from build123d import *

# Parameters (mm, degrees)
ESQUISSE3_R        = 9
BOSS_EXTRU_1_DEPTH = 5
ESQUISSE4_W        = 10
ESQUISSE4_H        = 3
ESQUISSE4_W_2      = 35
BOSS_EXTRU_2_DEPTH = 20


with BuildPart() as part:
    # Esquisse3 → Boss.-Extru.1 (new body)
    with BuildSketch(Plane(origin=(0, 0, 0), x_dir=(1, 0, 0), z_dir=(0, 1, 0))):
        with BuildLine():
            Line((-42.049920388, -18.295081967), (-42.049920388, 31.704918033))
            ThreePointArc((-42.049920388, 31.704918033), (-39.120988199, 38.775985845), (-32.049920388, 41.704918033))
            Line((-32.049920388, 41.704918033), (17.950079612, 41.704918033))
            ThreePointArc((17.950079612, 41.704918033), (25.021147424, 38.775985845), (27.950079612, 31.704918033))
            Line((27.950079612, 31.704918033), (27.950079612, -15.295081967))
            Line((27.950079612, -15.295081967), (52.950079612, -15.295081967))
            Line((52.950079612, -15.295081967), (52.950079612, -18.295081967))
            Line((52.950079612, -18.295081967), (17.950079612, -18.295081967))
            Line((17.950079612, -18.295081967), (17.950079612, 11.704918033))
            Line((17.950079612, 11.704918033), (-32.049920388, 11.704918033))
            Line((-32.049920388, 11.704918033), (-32.049920388, -18.295081967))
            Line((-32.049920388, -18.295081967), (-42.049920388, -18.295081967))
        make_face()
        with Locations((-20.049920388, 26.704918033)):
            Circle(ESQUISSE3_R, mode=Mode.SUBTRACT)
        with Locations((5.950079612, 26.704918033)):
            Circle(ESQUISSE3_R, mode=Mode.SUBTRACT)
    extrude(amount=BOSS_EXTRU_1_DEPTH)

    # Esquisse4 → Boss.-Extru.2 (add)
    with BuildSketch(Plane(origin=(0, 5, 0), x_dir=(1, 0, 0), z_dir=(0, 1, 0))):
        with Locations((-37.049920388, -16.795081967)):
            Rectangle(ESQUISSE4_W, ESQUISSE4_H)
        with Locations((35.450079612, -16.795081967)):
            Rectangle(ESQUISSE4_W_2, ESQUISSE4_H)
    extrude(amount=-BOSS_EXTRU_2_DEPTH)


solid = part.part
Input: part model. Units: mm. Frame: model coordinates. A direction names the side the tool comes from. Round coordinates to 2 decimals unless told otherwise and drop trailing zeros. Write each loop counter-clockwise with the first axis right and the second up, starting at its lowest first coordinate (ties: lowest second). Pieces come first, ordered by that corner, then holes.
1) Ray query, L1, parallel to X at y = 3.25, z = -6.5; L2, parallel to Y at x = -11, z = -27.5; L3, parallel to Z at x = 29.5, y = -4.5. Return the intervals inside material, ascending.
2) Contact query for flat-ended pins moving along their axis: P1, Ø8, axis at x = -35.5, y = -5.5, coming from the -Z side; P2, Ø5, axis at y = 2.5, z = 3, coming from the +X side; P3, Ø4, axis at x = -1.5, y = 1.5, coming from the +Z side. Output: stop coordinate, or through.
3) Cut plane A-A (y = -6.25). Return the cut outline in (x, z).
4) Cut plane D-D (x = 26). Return the cut outline in (y, z).
5) Cut plane B-B (z = 5.5). Return the cut outline in (x, y), then the cut area to 3 significant figures.
6) Cut plane C-C (y = 1). Return the cut outline in (x, z).
7) Draft query along X for faces 4 (the flat face through (17.95, 1, 6)), 5 (the flat face through (-37, -7, 15.295)), 6 (the flat face through (27.95, 2, -9)). Return one class per face: pulls with the +X half, pulls with the -X half, needs draft (parallel to the pull), parting line crosses it, or undercut.
8) Reachability of faces 1 (the flat face through (-32.05, 0.2, 6.7)), 2 (the flat face through (-37, -5, 18.295)), 3 (the flat face through (-7, 0, -20)) from +Z, -Z, +X, -X, +Y, -Y: full face, straight path, thin tool, end or side. Return the list, or none.
Geometry says:
1. L1: x = -42.05 to -32.05, 17.95 to 27.95
1. L2: y = 0 to 5
1. L3: z = 15.3 to 18.3
2. P1: stops at z = 15.3
2. P2: stops at x = 27.95
2. P3: stops at z = -11.7
3. outline: (-42.05, 15.3) - (-32.05, 15.3) - (-32.05, 18.3) - (-42.05, 18.3) - close; (17.95, 15.3) - (52.95, 15.3) - (52.95, 18.3) - (17.95, 18.3) - close
4. outline: (-15, 15.3) - (0, 15.3) - (0, -37.64) - (5, -37.64) - (5, 18.3) - (-15, 18.3) - close
5. outline: (-42.05, 0) - (-32.05, 0) - (-32.05, 5) - (-42.05, 5) - close; (17.95, 0) - (27.95, 0) - (27.95, 5) - (17.95, 5) - close
5. area: 100 mm2
6. outline: (-42.05, -31.7) arc R10 ccw to (-32.05, -41.7) - (17.95, -41.7) arc R10 ccw to (27.95, -31.7) - (27.95, 15.3) - (52.95, 15.3) - (52.95, 18.3) - (17.95, 18.3) - (17.95, -11.7) - (-32.05, -11.7) - (-32.05, 18.3) - (-42.05, 18.3) - close; hole circle Ø18 at (-20.05, -26.7); hole circle Ø18 at (5.95, -26.7)
7. face 4: undercut
7. face 5: needs draft
7. face 6: pulls with the +X half
8. face 1: +Z, +Y, -Y
8. face 2: +Z, +X, -X, +Y, -Y
8. face 3: -Z, +X, -X, -Y
